Part model, mm, in its own coordinate system. A direction names the side the tool comes from. Give positions to 0.01 mm unless a question says otherwise; leave off trailing zeros. Write each loop counter-clockwise with the first axis right and the second up, starting at its lowest first coordinate (ties: lowest second). Pieces come first, ordered by that corner, then holes. Notation, with made-up numbers: M -17,-27.75 L 1,-27.75 A20 ccw 1,7.25 Z; hole C 1.5,65 d5. An arc over 180 degrees is marked long. Use a Markdown table: item, result.
```python
from build123d import *

# Parameters (mm, degrees)
SKETCH1_W           = 250
SKETCH1_H           = 75
BOSS_EXTRUDE1_DEPTH = 15
BOSS_EXTRUDE2_DEPTH = 37.5
BOSS_EXTRUDE3_DEPTH = 75
CUT_EXTRUDE1_DEPTH  = 75


with BuildPart() as part:
    # Sketch1 → Boss-Extrude1 (new body)
    with BuildSketch(Plane(origin=(0, 0, 0), x_dir=(1, 0, 0), z_dir=(0, 1, 0))):
        Rectangle(SKETCH1_W, SKETCH1_H)
    extrude(amount=BOSS_EXTRUDE1_DEPTH)

    # Sketch3 → Boss-Extrude2 (add)
    with BuildSketch(Plane.XY):
        with BuildLine():
            Line((125, 15), (125, 35))
            ThreePointArc((125, 35), (98.074175964, 29.814560089), (75, 15))
            Line((75, 15), (125, 15))
        make_face()
    boss_extrude2 = extrude(amount=BOSS_EXTRUDE2_DEPTH)

    # Mirror1: Boss-Extrude2 across plane
    add(boss_extrude2.mirror(Plane(origin=(125, -37.5, 0), x_dir=(1, 0, 0), z_dir=(0, 0, 1))))

    # Sketch6 → Boss-Extrude3 (add)
    with BuildSketch(Plane.XY.offset(37.5)):
        Polygon((-125, 0), (-125, 15), (-156.545603012, 46.545603012), (-156.545603012, 31.545603012), align=None)
    extrude(amount=-BOSS_EXTRUDE3_DEPTH)

    # Sketch7 → Cut-Extrude1 (cut)
    with BuildSketch(Plane(origin=(-55, -55, 0), x_dir=(0, 0, -1), z_dir=(0.7071067811865438, 0.7071067811865513, 0))):
        Polygon((-37.5, 98.994949366), (-7.5, 143.607168979), (-37.5, 143.607168979), align=None)
        Polygon((7.5, 143.607168979), (37.5, 98.994949366), (37.5, 143.607168979), align=None)
    extrude(amount=-CUT_EXTRUDE1_DEPTH, mode=Mode.SUBTRACT)


solid = part.part
```
1. Cut at D-D, the plane x = 1. Give the cut face in (y, z).
Findings below:
| item | result |
|---|---|
| outline | M 0,-37.5 L 15,-37.5 L 15,37.5 L 0,37.5 Z |
2. Cut at B-B, the plane z = -19. Give the cut face in (x, y), then the cut area to 3 significant figures.
Findings below:
| item | result |
|---|---|
| outline | M -151.95,26.95 L -125,0 L 125,0 L 125,35 A72.5 ccw 75,15 L -125,15 L -144.45,34.45 Z |
| area | 4,790 mm2 |
3. Cut at A-A, the plane y = 23. Give the cut face in (x, z).
Findings below:
| item | result |
|---|---|
| outline | M -148,-22.76 L -133,-29.89 L -133,29.89 L -148,22.76 Z; M 85.05,-37.5 L 125,-37.5 L 125,37.5 L 85.05,37.5 Z |
4. Drop flat-ended pins along their axis: P1, Ø2, axis at y = 18, z = -10, coming from the -X side; P2, Ø1.5, axis at y = 17.5, z = 29.5, coming from the -X side; P3, Ø12, axis at x = -14.5, z = -7, coming from the +Y side. Give the stop position or say it passes through.
Findings below:
| item | result |
|---|---|
| P1 | x = -144 |
| P2 | x = -141.07 |
| P3 | y = 15 |
5. Tool access for faces 4 (the flat face through (-137, 27, 1)), 5 (the flat face through (-2, 0, -1)): list every direction of +Z, -Z, +X, -X, +Y, -Y with a clear straight run to the whole face (end or side of a thin tool).
Findings below:
| item | result |
|---|---|
| face 4 | +Z, -Z, +Y |
| face 5 | +Z, -Z, +X, -X, -Y |
6. Two-plate mould, pull along X, no slides. Class faces 1 (the flat face through (-137, 12, 1)), 2 (the flat face through (-6, 10, -37.5)), 3 (the cylindrical face through (98.433, 29.957, 0.525)): released by +X, released by -X, zero draft, split by the parting line, or undercut.
Findings below:
| item | result |
|---|---|
| face 1 | released by -X |
| face 2 | zero draft |
| face 3 | undercut |
7. Cut at C-C, the plane y = 4.5. Give the cut face in (x, z).
Findings below:
| item | result |
|---|---|
| outline | M -129.5,-37.5 L 125,-37.5 L 125,37.5 L -129.5,37.5 Z |
8. Drill centre lines: L1, parallel to Y at x = -120.5, z = 2; L2, parallel to X at y = 7.5, z = 32; L3, parallel to X at y = 22, z = 23. Where is each one in solid material? Low to high.
Findings below:
| item | result |
|---|---|
| L1 | 0 to 15 |
| L2 | -132.5 to 125 |
| L3 | -147 to -132, 83.58 to 125 |
